```python
from build123d import *

# Parameters (mm, degrees)
CROQUIS1_R               = 45
CROQUIS1_R_2             = 32.5
SALIENTE_EXTRUIR1_DEPTH  = 30
SALIENTE_EXTRUIR2_DEPTH  = 30
CROQUIS3_W               = 60
CROQUIS3_H               = 15
SALIENTE_EXTRUIR3_DEPTH  = 15
REDONDEO1_R              = 10
REDONDEO2_R              = 15
CROQUIS4_R               = 5
CORTAR_EXTRUIR1_DEPTH    = 16
REDONDEO1_OF_SIMETR_A1_R = 10
REDONDEO2_OF_SIMETR_A1_R = 15
CROQUIS8_R               = 6.25
SALIENTE_EXTRUIR4_DEPTH  = 11.25
SALIENTE_EXTRUIR5_START  = 10
SALIENTE_EXTRUIR5_DEPTH  = 20
CORTAR_EXTRUIR2_DEPTH    = 61
CROQUIS12_R              = 38
CROQUIS12_R_2            = 32.5
SALIENTE_EXTRUIR7_DEPTH  = 20
SALIENTE_EXTRUIR9_DEPTH  = 30


with BuildPart() as part:
    # Croquis1 → Saliente-Extruir1 (new body)
    with BuildSketch(Plane.XY):
        Circle(CROQUIS1_R)
        Circle(CROQUIS1_R_2, mode=Mode.SUBTRACT)
    extrude(amount=SALIENTE_EXTRUIR1_DEPTH)

    # Croquis2 → Saliente-Extruir2 (add)
    with BuildSketch(Plane.XY):
        with BuildLine():
            Line((-15, -42.426406871), (-15, -77.426406871))
            Line((-15, -77.426406871), (15, -77.426406871))
            Line((15, -77.426406871), (15, -42.426406871))
            ThreePointArc((15, -42.426406871), (0, -45), (-15, -42.426406871))
        make_face()
    saliente_extruir2 = extrude(amount=SALIENTE_EXTRUIR2_DEPTH)

    # Croquis3 → Saliente-Extruir3 (add, symmetric)
    with BuildSketch(Plane(origin=(0, 0, 0), x_dir=(0, 0, -1), z_dir=(1, 0, 0))):
        with Locations((-30, -69.926406871)):
            Rectangle(CROQUIS3_W, CROQUIS3_H)
    saliente_extruir3 = extrude(amount=SALIENTE_EXTRUIR3_DEPTH, both=True)

    # Redondeo1
    redondeo1_edges = [part.edges().sort_by_distance(p)[0] for p in [
        (-15, -69.926406871, 60),
        (15, -69.926406871, 60),
    ]]
    fillet(redondeo1_edges, radius=REDONDEO1_R)

    # Redondeo2
    redondeo2_edges = [part.edges().sort_by_distance(p)[0] for p in [
        (0, -77.426406871, 0),
    ]]
    fillet(redondeo2_edges, radius=REDONDEO2_R)

    # Croquis4 → Cortar-Extruir1 (cut, through all)
    with BuildSketch(Plane(origin=(0, -62.426406871, 0), x_dir=(1, 0, 0), z_dir=(0, 1, 0))):
        with Locations((0, -45)):
            Circle(CROQUIS4_R)
    cortar_extruir1 = extrude(amount=-CORTAR_EXTRUIR1_DEPTH, mode=Mode.SUBTRACT)

    # Simetría1: Saliente-Extruir2, Saliente-Extruir3, Cortar-Extruir1 across plane
    add(saliente_extruir2.mirror(Plane.ZX))
    add(saliente_extruir3.mirror(Plane.ZX))
    add(cortar_extruir1.mirror(Plane.ZX), mode=Mode.SUBTRACT)

    # Redondeo1 of Simetría1
    redondeo1_of_simetr_a1_edges = [part.edges().sort_by_distance(p)[0] for p in [
        (-15, 69.926406871, 60),
        (15, 69.926406871, 60),
    ]]
    fillet(redondeo1_of_simetr_a1_edges, radius=REDONDEO1_OF_SIMETR_A1_R)

    # Redondeo2 of Simetría1
    redondeo2_of_simetr_a1_edges = [part.edges().sort_by_distance(p)[0] for p in [
        (0, 77.426406871, 0),
    ]]
    fillet(redondeo2_of_simetr_a1_edges, radius=REDONDEO2_OF_SIMETR_A1_R)



with BuildPart() as body_2:
    # Croquis8 → Saliente-Extruir4 (new body, symmetric)
    with BuildSketch(Plane(origin=(0, 0, 0), x_dir=(1, 0, 0), z_dir=(0, 1, 0))):
        with BuildLine():
            Line((-45, -30), (-70.006566453, -30))
            Line((-70.006566453, -30), (-103.60103907, -74.743636588))
            ThreePointArc((-103.60103907, -74.743636588), (-123.92378818, -85.155995163), (-119.59473224, -62.735232082))
            Line((-119.59473224, -62.735232082), (-80, -10))
            Line((-80, -10), (-45, -10))
            Line((-45, -10), (-45, -30))
        make_face()
        with Locations((-116.298451318, -75)):
            Circle(CROQUIS8_R, mode=Mode.SUBTRACT)
    extrude(amount=SALIENTE_EXTRUIR4_DEPTH, both=True)


with BuildPart() as part_1:
    add(part.part)

    add(body_2.part)  # Saliente-Extruir5 merges body 2
    # Croquis9 → Saliente-Extruir5 (add)
    with BuildSketch(Plane.XY.offset(SALIENTE_EXTRUIR5_START)):
        with BuildLine():
            Line((-43.571062645, 11.25), (-45, 11.25))
            Line((-45, 11.25), (-45, 0))
            ThreePointArc((-45, 0), (-44.641336332, 5.670193162), (-43.571062645, 11.25))
        make_face()
        with BuildLine():
            ThreePointArc((-43.571062645, -11.25), (-44.641336332, -5.670193162), (-45, 0))
            Line((-45, 0), (-45, -11.25))
            Line((-45, -11.25), (-43.571062645, -11.25))
        make_face()
    extrude(amount=SALIENTE_EXTRUIR5_DEPTH)

    # Croquis11 → Cortar-Extruir2 (cut, through all)
    with BuildSketch(Plane.ZY.offset(15)):
        with BuildLine():
            Line((0, 62.426406871), (0, 52.426406871))
            Line((0, 52.426406871), (25, 77.426406871))
            Line((25, 77.426406871), (15, 77.426406871))
            ThreePointArc((15, 77.426406871), (4.393398282, 73.033008589), (0, 62.426406871))
        make_face()
    cortar_extruir2 = extrude(amount=-CORTAR_EXTRUIR2_DEPTH, mode=Mode.SUBTRACT)

    # Simetría2: Cortar-Extruir2 across plane
    add(cortar_extruir2.mirror(Plane.ZX), mode=Mode.SUBTRACT)

    # Croquis12 → Saliente-Extruir7 (add)
    with BuildSketch(Plane(origin=(0, 0, 0), x_dir=(-1, 0, 0), z_dir=(0, 0, -1))):
        Circle(CROQUIS12_R)
        Circle(CROQUIS12_R_2, mode=Mode.SUBTRACT)
    extrude(amount=SALIENTE_EXTRUIR7_DEPTH)

    # Croquis13 → Saliente-Extruir9 (add)
    with BuildSketch(Plane.ZY.offset(15)):
        Polygon((30, 62.426406871), (30, 51.426406871), (41, 62.426406871), align=None)
    saliente_extruir9 = extrude(amount=-SALIENTE_EXTRUIR9_DEPTH)

    # Simetría3: Saliente-Extruir9 across plane
    add(saliente_extruir9.mirror(Plane.ZX))

    # Croquis14 → Revolución1 (revolve)
    with BuildSketch(Plane(origin=(0, 0, 0), x_dir=(0, 0, -1), z_dir=(1, 0, 0))):
        with BuildLine():
            Line((-49.5, 77.426406871), (-49.5, 92.426406871))
            ThreePointArc((-49.5, 92.426406871), (-51.757815193, 103.348424917), (-42.5, 109.5678353))
            Line((-42.5, 109.5678353), (-42.5, 77.426406871))
            Line((-42.5, 77.426406871), (-49.5, 77.426406871))
        make_face()
    revoluci_n1 = revolve(axis=Axis((0, 77.426406871, 42.5), (0, 1, 0)))

    # Simetría4: Revolución1 across plane
    add(revoluci_n1.mirror(Plane.ZX))


solid = part_1.part
```
Verification items for the finished model (mm, model axes). A direction names the side the tool comes from. Coordinates: 2 decimals unless noted, no trailing zeros. Loops run counter-clockwise (first coordinate to the right, second up) from the corner with the lowest first, then second, coordinate; pieces in that order, holes last. Notation, with made-up numbers: (-20.75, 66.5) -> (25.25, 66.5) arc R22 ccw to (25.25, 100.5) -> close; hole circle Ø6 at (5.5, 43.5). An arc over 180 degrees is marked (long way). Answer in a Markdown table with one row per item.
1) Access from +Z, -Z, +X, -X, +Y, -Y to the whole of each face (thin tool, end or side, straight path). Record for faces 5 (the face through (-27, -27, 0)), 6 (the face through (2.103, 85.031, 49.177)), 7 (the face through (-0.21, -56.849, 35.423)).
The answers:
| item | result |
|---|---|
| face 5 | -Z |
| face 6 | none |
| face 7 | +Z, +X, -X |
2) Section check D-D (y = 65.5). Record the cut outline in (x, z).
The answers:
| item | result |
|---|---|
| outline | (-15, 13.07) -> (15, 13.07) -> (15, 50) arc R10 ccw to (5, 60) -> (-5, 60) arc R10 ccw to (-15, 50) -> close; hole circle Ø10 at (0, 45) |
3) Section check C-C (x = 28.5). Record the cut outline in (y, z).
The answers:
| item | result |
|---|---|
| outline | (-34.82, 0) -> (-25.13, 0) -> (-25.13, -20) -> (-15.62, -20) -> (-15.62, 30) -> (-34.82, 30) -> close; (15.62, -20) -> (25.13, -20) -> (25.13, 0) -> (34.82, 0) -> (34.82, 30) -> (15.62, 30) -> close |
4) Scan lines: line 1 along X through (y, z) = (73.75, 45); line 2 along X through (y, z) = (-1, 75); line 3 along Y through (x, z) = (-97.5, 62.5). Record each from-to range of solid material in increasing order. Write a range as from..to.
The answers:
| item | result |
|---|---|
| line 1 | x = -15..-5, 5..15 |
| line 2 | x = -129..-122.55, -110.05..-103.6 |
| line 3 | y = -11.25..11.25 |
5) Draft check along X on faces 1 (the face through (0, 77.426, 45)), 2 (the face through (15, 60, 25)), 3 (the face through (-86, 11.25, 40)), 4 (the face through (-17.535, -33.713, -9.86)). Enter one of: released by +X, released by -X, zero draft, split by the parting line, or undercut.
The answers:
| item | result |
|---|---|
| face 1 | undercut |
| face 2 | released by +X |
| face 3 | zero draft |
| face 4 | split by the parting line |
6) Section check B-B (z = 45). Record the cut outline in (x, y), and give its area (3 significant figures).
The answers:
| item | result |
|---|---|
| outline | (-106.28, -11.25) -> (-81.27, -11.25) -> (-81.27, 11.25) -> (-106.28, 11.25) -> close; (-15, -77.43) -> (-6.54, -77.43) -> (-6.54, -92.43) arc R9.68 ccw (long way) to (6.54, -92.43) -> (6.54, -77.43) -> (15, -77.43) -> (15, -62.43) -> (5, -62.43) -> (5, -77.43) -> (-5, -77.43) -> (-5, -62.43) -> (-15, -62.43) -> close; (-15, 62.43) -> (-5, 62.43) -> (-5, 77.43) -> (5, 77.43) -> (5, 62.43) -> (15, 62.43) -> (15, 77.43) -> (6.54, 77.43) -> (6.54, 92.43) arc R9.68 ccw (long way) to (-6.54, 92.43) -> (-6.54, 77.43) -> (-15, 77.43) -> close |
| area | 2,100 mm2 |
7) Section check A-A (y = 0). Record the cut outline in (x, z).
The answers:
| item | result |
|---|---|
| outline | (-119.59, 62.74) -> (-80, 10) -> (-45, 10) -> (-45, 0) -> (-38, 0) -> (-38, -20) -> (-32.5, -20) -> (-32.5, 30) -> (-70.01, 30) -> (-103.6, 74.74) arc R12.7 ccw (long way) to start; (32.5, -20) -> (38, -20) -> (38, 0) -> (45, 0) -> (45, 30) -> (32.5, 30) -> close; hole circle Ø12.5 at (-116.3, 75) |
8) Depth check by flat-ended pin: P1, Ø4, axis at y = -28.5, z = 29.5, coming from the +X side; P2, Ø10, axis at x = -55, y = 6, coming from the -Z side; P3, Ø5, axis at x = 2, z = 29, coming from the +Y side. Enter the tip coordinate at first touch or a pass-through.
The answers:
| item | result |
|---|---|
| P1 | stops at x = 36.37 |
| P2 | stops at z = 10 |
| P3 | stops at y = 77.43 |
